Input: part model. Units: mm. Frame: model coordinates. Face numbers are marked on the shaded views. Coordinates: 2 decimals unless noted, no trailing zeros. Order: outer loops, then holes, each group sorted by start corner. A loop starts at its lowest first (then second) coordinate and runs counter-clockwise, first axis right, second up. Notation, with made-up numbers: (-11, 88.5) -> (41, 88.5) arc R19 cw to (41, 124.5) -> close; hole circle Ø4 at (67.25, 17.25). An arc over 180 degrees is marked (long way). Write each question's results on one line, items separated by ' | '.
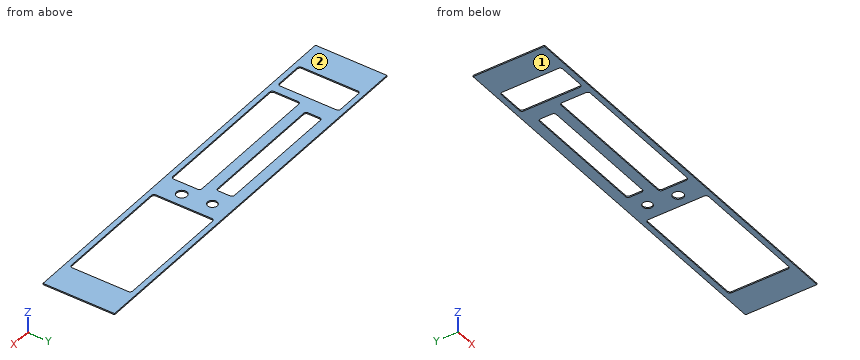
```python
from build123d import *

# Parameters (mm, degrees)
SKETCH1_W           = 482.6
SKETCH1_H           = 88.0999
BOSS_EXTRUDE1_DEPTH = 1.5875
SKETCH2_W           = 158.496
SKETCH2_H           = 20.574
CUT_EXTRUDE1_DEPTH  = 246.292902978
FILLET1_R           = 3.175
SKETCH3_W           = 177.8
SKETCH3_H           = 35.7759
CUT_EXTRUDE2_DEPTH  = 246.292902978
FILLET2_R           = 3.175
SKETCH4_W           = 38.1
SKETCH4_H           = 75.3999
CUT_EXTRUDE3_DEPTH  = 246.292902978
SKETCH5_W           = 147.96262
SKETCH5_H           = 75.3999
CUT_EXTRUDE4_DEPTH  = 1.5875
FILLET3_R           = 3.175
SKETCH6_R           = 6.5024
SKETCH6_R_2         = 5.92074
CUT_EXTRUDE5_DEPTH  = 246.292902978


with BuildPart() as part:
    # Sketch1 → Boss-Extrude1 (new body)
    with BuildSketch(Plane.XY):
        Rectangle(SKETCH1_W, SKETCH1_H)
    extrude(amount=BOSS_EXTRUDE1_DEPTH)

    # Sketch2 → Cut-Extrude1 (cut, through all)
    with BuildSketch(Plane.XY.offset(1.5875)):
        with Locations((-65.41262, 21.06295)):
            Rectangle(SKETCH2_W, SKETCH2_H)
    extrude(amount=-CUT_EXTRUDE1_DEPTH, mode=Mode.SUBTRACT)

    # Fillet1
    fillet1_edges = [part.edges().sort_by_distance(p)[0] for p in [
        (-144.66062, 10.77595, 0.79375),
        (-144.66062, 31.34995, 0.79375),
        (13.83538, 31.34995, 0.79375),
        (13.83538, 10.77595, 0.79375),
    ]]
    fillet(fillet1_edges, radius=FILLET1_R)

    # Sketch3 → Cut-Extrude2 (cut, through all)
    with BuildSketch(Plane.XY.offset(1.5875)):
        with Locations((-65.41262, -19.812)):
            Rectangle(SKETCH3_W, SKETCH3_H)
    extrude(amount=-CUT_EXTRUDE2_DEPTH, mode=Mode.SUBTRACT)

    # Fillet2
    fillet2_edges = [part.edges().sort_by_distance(p)[0] for p in [
        (-154.31262, -37.69995, 0.79375),
        (-154.31262, -1.92405, 0.79375),
        (23.48738, -1.92405, 0.79375),
        (23.48738, -37.69995, 0.79375),
    ]]
    fillet(fillet2_edges, radius=FILLET2_R)

    # Sketch4 → Cut-Extrude3 (cut, through all)
    with BuildSketch(Plane.XY.offset(1.5875)):
        with Locations((-184.15, 0)):
            Rectangle(SKETCH4_W, SKETCH4_H)
    extrude(amount=-CUT_EXTRUDE3_DEPTH, mode=Mode.SUBTRACT)

    # Sketch5 → Cut-Extrude4 (cut)
    with BuildSketch(Plane.XY.offset(1.5875)):
        with Locations((129.21869, 0)):
            Rectangle(SKETCH5_W, SKETCH5_H)
    extrude(amount=-CUT_EXTRUDE4_DEPTH, mode=Mode.SUBTRACT)

    # Fillet3
    fillet3_edges = [part.edges().sort_by_distance(p)[0] for p in [
        (-203.2, -37.69995, 0.79375),
        (-203.2, 37.69995, 0.79375),
        (-165.1, 37.69995, 0.79375),
        (-165.1, -37.69995, 0.79375),
        (55.23738, -37.69995, 0.79375),
        (55.23738, 37.69995, 0.79375),
        (203.2, 37.69995, 0.79375),
        (203.2, -37.69995, 0.79375),
    ]]
    fillet(fillet3_edges, radius=FILLET3_R)

    # Sketch6 → Cut-Extrude5 (cut, through all)
    with BuildSketch(Plane(origin=(0, 0, 0), x_dir=(-1, 0, 0), z_dir=(0, 0, -1))):
        with Locations((-39.36238, -13.56995)):
            Circle(SKETCH6_R)
        with Locations((-34.93008, 21.14042)):
            Circle(SKETCH6_R_2)
    extrude(amount=-CUT_EXTRUDE5_DEPTH, mode=Mode.SUBTRACT)


solid = part.part
```
(1) Cut plane C-C, the plane z = 1.2. Count the separate pieces of the cut face and the enclosed holes in it, plus the area to 3 significant figures.
Return value:
separate pieces: 1 | enclosed holes: 6 | area: 18,700 mm2
(2) Cut plane A-A, the plane x = 86.5. Return loops of the section in (y, z).
Return value:
outline: (-44.05, 0) -> (-37.7, 0) -> (-37.7, 1.59) -> (-44.05, 1.59) -> close; (37.7, 0) -> (44.05, 0) -> (44.05, 1.59) -> (37.7, 1.59) -> close
(3) Line query: line 1 along X through (y, z) = (20.5, 1.4); line 2 along X through (y, z) = (1.5, 1); line 3 along X through (y, z) = (-30, 0.1). Output: solid intervals per line, ascending. Write a range as from..to.
Return value:
line 1: -241.3..-203.2, -165.1..-144.66, 13.84..29.04, 40.82..55.24, 203.2..241.3 | line 2: -241.3..-203.2, -165.1..55.24, 203.2..241.3 | line 3: -241.3..-203.2, -165.1..-154.31, 23.49..55.24, 203.2..241.3
(4) Cut plane B-B, the plane x = -27. Return loops of the section in (y, z), plus the area to 3 significant figures.
Return value:
outline: (-44.05, 0) -> (-37.7, 0) -> (-37.7, 1.59) -> (-44.05, 1.59) -> close; (-1.92, 0) -> (10.78, 0) -> (10.78, 1.59) -> (-1.92, 1.59) -> close; (31.35, 0) -> (44.05, 0) -> (44.05, 1.59) -> (31.35, 1.59) -> close | area: 50.4 mm2
(5) Pin query (flat end, axial travel): P1, Ø7, axis at x = 34.93, y = 21.14, coming from the -Z side. Return the tip coordinate at first contact, or that it passes through.
Return value:
P1: through
(6) Mould query, pull axis Z, two halves, no side actions, for the marked faces 1 and 2. Classes: +Z half, -Z half, draft (parallel to the pull), parting line (faces both ways), or undercut.
Return value:
face 1: -Z half | face 2: +Z half
